```python
from build123d import *

# Parameters (mm, degrees)
ESQUISSE1_W             = 125
ESQUISSE1_H             = 55
BOSS_EXTRU_3_DEPTH      = 5
ESQUISSE2_R             = 3.5
ENL_V_MAT_EXTRU_1_DEPTH = 5
ESQUISSE3_W             = 4.868398839
ESQUISSE3_H             = 10
ESQUISSE3_W_2           = 5
ESQUISSE3_W_3           = 12.5
ESQUISSE3_H_2           = 5
ESQUISSE3_W_4           = 15
ENL_V_MAT_EXTRU_2_DEPTH = 5
ESQUISSE4_R             = 1.5
ENL_V_MAT_EXTRU_3_DEPTH = 2.5
ESQUISSE5_R             = 1.5
ENL_V_MAT_EXTRU_4_DEPTH = 77.546049734


with BuildPart() as part:
    # Esquisse1 → Boss.-Extru.3 (new body)
    with BuildSketch(Plane.XY):
        with Locations((-4.111168033, 9.879807692)):
            Rectangle(ESQUISSE1_W, ESQUISSE1_H)
    extrude(amount=BOSS_EXTRU_3_DEPTH)

    # Esquisse2 → Enlèv. mat.-Extru.1 (cut)
    with BuildSketch(Plane.XY.offset(5)):
        with Locations((-4.111168033, 9.879807692)):
            Circle(ESQUISSE2_R)
    extrude(amount=-ENL_V_MAT_EXTRU_1_DEPTH, mode=Mode.SUBTRACT)

    # Esquisse3 → Enlèv. mat.-Extru.2 (cut)
    with BuildSketch(Plane.XY.offset(5)):
        with Locations((50.954632547, 17.379807692)):
            Rectangle(ESQUISSE3_W, ESQUISSE3_H)
        with Locations((50.888831967, -2.620192308)):
            Rectangle(ESQUISSE3_W_2, ESQUISSE3_H)
        with Locations((-59.111168033, 17.379807692)):
            Rectangle(ESQUISSE3_W_2, ESQUISSE3_H)
        with Locations((-59.111168033, -2.620192308)):
            Rectangle(ESQUISSE3_W_2, ESQUISSE3_H)
        with Locations((-47.861168033, 29.879807692)):
            Rectangle(ESQUISSE3_W_3, ESQUISSE3_H_2)
        with Locations((-19.111168033, 29.879807692)):
            Rectangle(ESQUISSE3_W_4, ESQUISSE3_H_2)
        with Locations((10.888831967, 29.879807692)):
            Rectangle(ESQUISSE3_W_4, ESQUISSE3_H_2)
        with Locations((39.638831967, 29.879807692)):
            Rectangle(ESQUISSE3_W_3, ESQUISSE3_H_2)
    extrude(amount=-ENL_V_MAT_EXTRU_2_DEPTH, mode=Mode.SUBTRACT)

    # Esquisse4 → Enlèv. mat.-Extru.3 (cut)
    with BuildSketch(Plane.XY.offset(5)):
        with Locations((-46.611168033, 9.879807692)):
            Circle(ESQUISSE4_R)
        with Locations((38.388831967, 9.879807692)):
            Circle(ESQUISSE4_R)
    extrude(amount=-ENL_V_MAT_EXTRU_3_DEPTH, mode=Mode.SUBTRACT)

    # Esquisse5 → Enlèv. mat.-Extru.4 (cut, through all)
    with BuildSketch(Plane.XY.offset(5)):
        with Locations((4.388831967, 9.879807692)):
            Circle(ESQUISSE5_R)
        with Locations((-12.611168033, 9.879807692)):
            Circle(ESQUISSE5_R)
    extrude(amount=-ENL_V_MAT_EXTRU_4_DEPTH, mode=Mode.SUBTRACT)


solid = part.part
```
CAD build for the part. Positions are in the model's coordinates, mm. A direction names the side the tool comes from. Round coordinates to 2 decimals unless told otherwise and drop trailing zeros. Loops run counter-clockwise (first coordinate to the right, second up) from the corner with the lowest first, then second, coordinate; pieces in that order, holes last. Notation, with made-up numbers: M 26.25,81.5 L 42.25,81.5 A32 cw 42.25,119.5 Z; hole C 37,-10 d4. An arc over 180 degrees is marked long. Use a Markdown table: item, result. Add a question column.
(1) Pull direction Y, two halves, no side cores. Call faces 4 (the face through (51, 22.38, 3)), 5 (the face through (-5, -17.62, 2)), 6 (the face through (-5, 4, 0)): +Y half, -Y half, draft (parallel to the pull), parting line (faces both ways), or undercut.
(2) Cut at B-B (y = 28.5). Give the cut face in (x, z).
(3) Cut at A-A (x = -25). Give the cut face in (y, z).
(4) Cut at C-C (z = 4). State how many separate pieces and enclosed holes the cut face has, and give its area (3 significant figures).
(5) Drill centre lines: line 1 (X direction, y = -3, z = 4.05); line 2 (X direction, y = 16, z = 3.75); line 3 (Y direction, x = -58, z = 0.7). Where is each one in solid material? Low to high.
(6) Which spindle directions (+Z, -Z, +X, -X, +Y, -Y) get a long thin tool onto all of the face, cutting with end or side? Do faces 1 (the face through (11, 27.38, 3)), 2 (the face through (-5, 37.38, 2)), 3 (the face through (38, 10, 2.5)). Say none if no direction does.
Geometry says:
| question | item | result |
|---|---|---|
| 1 | face 4 | undercut |
| 1 | face 5 | -Y half |
| 1 | face 6 | draft |
| 2 | outline | M -66.61,0 L -54.11,0 L -54.11,5 L -66.61,5 Z; M -41.61,0 L -26.61,0 L -26.61,5 L -41.61,5 Z; M -11.61,0 L 3.39,0 L 3.39,5 L -11.61,5 Z; M 18.39,0 L 33.39,0 L 33.39,5 L 18.39,5 Z; M 45.89,0 L 58.39,0 L 58.39,5 L 45.89,5 Z |
| 3 | outline | M -17.62,0 L 27.38,0 L 27.38,5 L -17.62,5 Z; M 32.38,0 L 37.38,0 L 37.38,5 L 32.38,5 Z |
| 4 | separate pieces | 1 |
| 4 | enclosed holes | 13 |
| 4 | area | 6,330 mm² |
| 5 | line 1 | x = -66.61 to -61.61, -56.61 to 48.39, 53.39 to 58.39 |
| 5 | line 2 | x = -66.61 to -61.61, -56.61 to 48.52, 53.39 to 58.39 |
| 5 | line 3 | y = -17.62 to -7.62, 2.38 to 12.38, 22.38 to 37.38 |
| 6 | face 1 | +Z, -Z |
| 6 | face 2 | +Z, -Z, +X, -X, +Y |
| 6 | face 3 | +Z |
